```python
from build123d import *

# Parameters (mm, degrees)
SKETCH1_R           = 160.85
SKETCH1_R_2         = 3.556
SKETCH1_R_3         = 148.15
BOSS_EXTRUDE1_DEPTH = 5.08
SKETCH2_R           = 168.275
SKETCH2_R_2         = 160.85
BOSS_EXTRUDE2_DEPTH = 2.54
CUT_EXTRUDE1_DEPTH  = 6.08


with BuildPart() as part:
    # Sketch1 → Boss-Extrude1 (new body)
    with BuildSketch(Plane(origin=(0, 0, 0), x_dir=(1, 0, 0), z_dir=(0, 1, 0))):
        Circle(SKETCH1_R)
        with Locations((0, 154.5)):
            Circle(SKETCH1_R_2, mode=Mode.SUBTRACT)
        with Locations((133.800924885, 77.25)):
            Circle(SKETCH1_R_2, mode=Mode.SUBTRACT)
        with Locations((133.800924885, -77.25)):
            Circle(SKETCH1_R_2, mode=Mode.SUBTRACT)
        with Locations((0, -154.5)):
            Circle(SKETCH1_R_2, mode=Mode.SUBTRACT)
        with Locations((-133.800924885, -77.25)):
            Circle(SKETCH1_R_2, mode=Mode.SUBTRACT)
        with Locations((-133.800924885, 77.25)):
            Circle(SKETCH1_R_2, mode=Mode.SUBTRACT)
        Circle(SKETCH1_R_3, mode=Mode.SUBTRACT)
    extrude(amount=BOSS_EXTRUDE1_DEPTH)

    # Sketch2 → Boss-Extrude2 (add)
    with BuildSketch(Plane(origin=(0, 5.08, 0), x_dir=(1, 0, 0), z_dir=(0, 1, 0))):
        Circle(SKETCH2_R)
        Circle(SKETCH2_R_2, mode=Mode.SUBTRACT)
    extrude(amount=-BOSS_EXTRUDE2_DEPTH)

    # Sketch3 → Cut-Extrude1 (cut, through all)
    with BuildSketch(Plane(origin=(0, 5.08, 0), x_dir=(1, 0, 0), z_dir=(0, 1, 0))):
        with BuildLine():
            Line((-88.9, 153.979316793), (-84.1375, 145.730424822))
            ThreePointArc((-84.1375, 145.730424822), (-77.700747892, 149.261747953), (-71.116087994, 152.508942864))
            Line((-71.116087994, 152.508942864), (-66.863491736, 143.389220757))
            ThreePointArc((-66.863491736, 143.389220757), (-73.054402471, 140.336201444), (-79.10625, 137.016044196))
            Line((-79.10625, 137.016044196), (0, 0))
            Line((0, 0), (-79.10625, -137.016044196))
            ThreePointArc((-79.10625, -137.016044196), (-85.007514286, -133.435069121), (-90.746961936, -129.600092807))
            Line((-90.746961936, -129.600092807), (-96.518574827, -137.842810253))
            ThreePointArc((-96.518574827, -137.842810253), (-90.414091595, -141.921695544), (-84.1375, -145.730424822))
            Line((-84.1375, -145.730424822), (-88.9, -153.979316793))
            ThreePointArc((-88.9, -153.979316793), (177.8, 0), (-88.9, 153.979316793))
        make_face()
    extrude(amount=-CUT_EXTRUDE1_DEPTH, mode=Mode.SUBTRACT)


solid = part.part
```
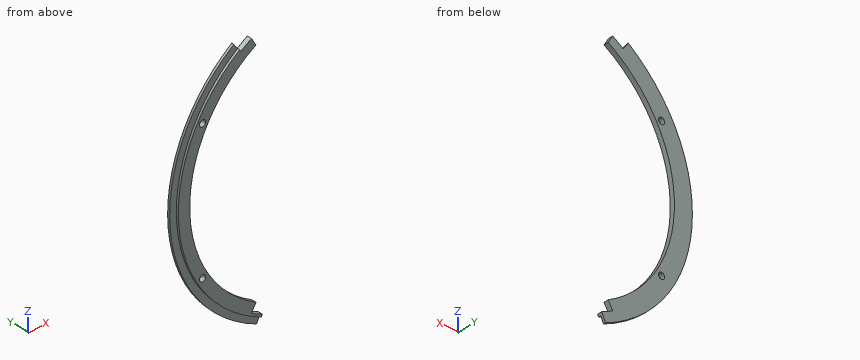
Part model, mm, in its own coordinate system. Round coordinates to 2 decimals unless told otherwise and drop trailing zeros. Loops run counter-clockwise (first coordinate to the right, second up) from the corner with the lowest first, then second, coordinate; pieces in that order, holes last. Notation, with made-up numbers: (-26.5, -32) -> (-0.5, -32) arc R18 cw to (-0.5, -9) -> close; hole circle Ø4 at (-16.75, -11). An arc over 180 degrees is marked (long way). Use CSV: the item, a comma, the result in double quotes. Start each with the question number.
1) Cut at A-A, the plane x = -140.5. Write the cut outline in (y, z), plus the area to 3 significant figures.
2) Cut at B-B, the plane y = 3.45. Give the number of separate pieces and of enclosed holes in the cut face, plus the area to 3 significant figures.
3) Cut at C-C, the plane z = 77.25. Write the cut outline in (x, y), plus the area to 3 significant figures.
4) Wall check: L1, parallel to Z at x = -137, y = 4.8; L2, parallel to Z at x = -115, y = 2; L3, parallel to Z at x = -81, y = 1.3. Give the ranges that are in metal, low to high. Write a range as [from, to].
5) Cut at D-D, the plane x = -105. Write the cut outline in (y, z), plus the area to 3 significant figures.
6) Drop flat-ended pins along their axis: P1, Ø1.5, axis at x = -109.5, y = 2.5, coming from the -Z side; P2, Ø3, axis at x = -122, y = 3, coming from the -Z side; P3, Ø3, axis at x = -141, y = 2, coming from the -Z side; P4, Ø5.5, axis at x = -133.8, z = 77.25, coming from the -Y side. Give the stop position or say it passes through.
Determined:
1,outline,"(0, -78.31) -> (2.54, -78.31) -> (2.54, -92.61) -> (5.08, -92.61) -> (5.08, -46.99) -> (0, -46.99) -> close; (0, 46.99) -> (5.08, 46.99) -> (5.08, 92.61) -> (2.54, 92.61) -> (2.54, 78.31) -> (0, 78.31) -> close"
1,area,"391 mm2"
2,separate pieces,"1"
2,enclosed holes,"2"
2,area,"6,590 mm2"
3,outline,"(-149.5, 2.54) -> (-141.09, 2.54) -> (-141.09, 0) -> (-137.36, 0) -> (-137.36, 5.08) -> (-149.5, 5.08) -> close; (-130.24, 0) -> (-126.42, 0) -> (-126.42, 5.08) -> (-130.24, 5.08) -> close"
3,area,"59.8 mm2"
4,L1,"z = [-97.71, -78.8], [-75.7, -56.39], [56.39, 75.7], [78.8, 97.71]"
4,L2,"z = [-112.46, -93.4], [93.4, 112.46]"
4,L3,"z = [-138.97, -124.05], [124.05, 135.91]"
5,outline,"(0, -121.85) -> (2.54, -121.85) -> (2.54, -131.5) -> (5.08, -131.5) -> (5.08, -104.52) -> (0, -104.52) -> close; (0, 104.52) -> (5.08, 104.52) -> (5.08, 131.5) -> (2.54, 131.5) -> (2.54, 121.85) -> (0, 121.85) -> close"
5,area,"225 mm2"
6,P1,"stops at z = -128.41"
6,P2,"stops at z = -117.46"
6,P3,"stops at z = -93.96"
6,P4,"passes through"
